```python
from build123d import *

# Parameters (mm, degrees)
CYLINDER_R           = 35
CYLINDER_DEPTH       = 100
CYLINDER_PITCH_ANGLE = 90
BOX003_W             = 170
BOX003_H             = 169
BOX003_DEPTH         = 74
BOX001_W             = 170
BOX001_H             = 190
BOX001_DEPTH         = 166
BOX_W                = 180
BOX_H                = 200
BOX_DEPTH            = 350
BOX002_W             = 180
BOX002_H             = 80
BOX002_DEPTH         = 28
FILLET_R             = 10
FILLET001_R          = 10
FILLET002_R          = 10
FILLET003_R          = 10
FILLET004_R          = 10
FILLET005_R          = 15
FILLET006_R          = 10


with BuildPart() as cylinder:
    # Cylinder → Cylinder (new body)
    with BuildSketch(Plane.XY):
        Circle(CYLINDER_R)
    extrude(amount=CYLINDER_DEPTH)


with BuildPart() as cylinder_1:
    # Cylinder pitch: moved
    add(cylinder.part.rotate(Axis((0, 0, 0), (0, 1, 0)), CYLINDER_PITCH_ANGLE))


with BuildPart() as cylinder_2:
    # Cylinder placement: moved
    add(cylinder_1.part.moved(Location((43, 100, 70))))


with BuildPart() as cube003:
    # Box003 → Box003 (new body)
    with BuildSketch(Plane(origin=(5, -68, 5), x_dir=(1, 0, 0), z_dir=(0, 0, 1))):
        with Locations((85, 84.5)):
            Rectangle(BOX003_W, BOX003_H)
    extrude(amount=BOX003_DEPTH)


with BuildPart() as cube001:
    # Box001 → Box001 (new body)
    with BuildSketch(Plane(origin=(5, 5, 187), x_dir=(1, 0, 0), z_dir=(0, 0, 1))):
        with Locations((85, 95)):
            Rectangle(BOX001_W, BOX001_H)
    extrude(amount=BOX001_DEPTH)


with BuildPart() as cone:
    # Cone → Cone (revolve)
    with BuildSketch(Plane(origin=(90, 100, 88), x_dir=(1, 0, 0), z_dir=(0, -1, 0))):
        Polygon((0, 0), (40, 0), (85, 100), (0, 100), align=None)
    revolve(axis=Axis((90, 100, 88), (0, 0, 1)))


with BuildPart() as cut001:
    # Box → Box (new body)
    with BuildSketch(Plane.XY):
        with Locations((90, 100)):
            Rectangle(BOX_W, BOX_H)
    extrude(amount=BOX_DEPTH)

    # Cut: cut Cone
    add(cone.part, mode=Mode.SUBTRACT)

    # Cut001: cut Cube001
    add(cube001.part, mode=Mode.SUBTRACT)


with BuildPart() as fillet006:
    # Box002 → Box002 (new body)
    with BuildSketch(Plane(origin=(0, -75, 0), x_dir=(1, 0, 0), z_dir=(0, 0, 1))):
        with Locations((90, 40)):
            Rectangle(BOX002_W, BOX002_H)
    extrude(amount=BOX002_DEPTH)

    # Fusion: union Cut001
    add(cut001.part)

    # Cut002: cut Cube003
    add(cube003.part, mode=Mode.SUBTRACT)

    # Cut003: cut Cylinder
    add(cylinder_2.part, mode=Mode.SUBTRACT)

    # Fillet
    fillet_edges = [fillet006.edges().sort_by_distance(p)[0] for p in [
        (180, 200, 175),
    ]]
    fillet(fillet_edges, radius=FILLET_R)

    # Fillet001
    fillet001_edges = [fillet006.edges().sort_by_distance(p)[0] for p in [
        (0, 200, 175),
    ]]
    fillet(fillet001_edges, radius=FILLET001_R)

    # Fillet002
    fillet002_edges = [fillet006.edges().sort_by_distance(p)[0] for p in [
        (180, -75, 14),
    ]]
    fillet(fillet002_edges, radius=FILLET002_R)

    # Fillet003
    fillet003_edges = [fillet006.edges().sort_by_distance(p)[0] for p in [
        (0, -75, 14),
    ]]
    fillet(fillet003_edges, radius=FILLET003_R)

    # Fillet004
    fillet004_edges = [fillet006.edges().sort_by_distance(p)[0] for p in [
        (5.45, 100, 187),
    ]]
    fillet(fillet004_edges, radius=FILLET004_R)

    # Fillet005
    fillet005_edges = [fillet006.edges().sort_by_distance(p)[0] for p in [
        (93, 101, 35.014289),
    ]]
    fillet(fillet005_edges, radius=FILLET005_R)

    # Fillet006
    fillet006_edges = [fillet006.edges().sort_by_distance(p)[0] for p in [
        (90, 0, 79),
    ]]
    fillet(fillet006_edges, radius=FILLET006_R)


solid = fillet006.part
```
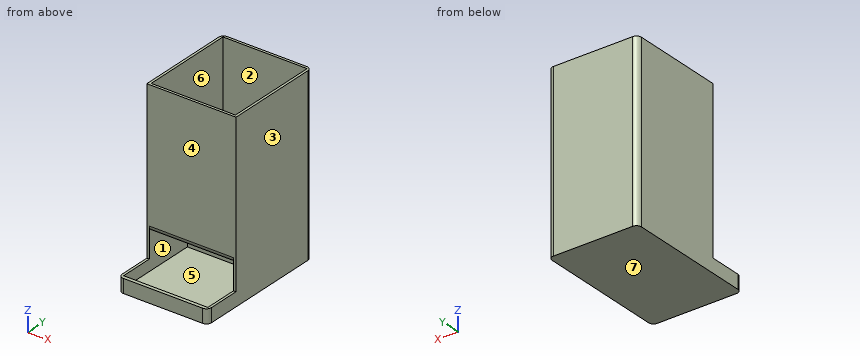
Could you check a few things on this model? Use its own coordinates, in mm. Face numbers are marked on the shaded views. A direction names the side the tool comes from. Give positions to 0.01 mm unless a question says otherwise; leave off trailing zeros. Loops run counter-clockwise (first coordinate to the right, second up) from the corner with the lowest first, then second, coordinate; pieces in that order, holes last. Notation, with made-up numbers: (65, 65.25) -> (107, 65.25) arc R11 cw to (107, 74.25) -> close; hole circle Ø4 at (-18, 67.25). An arc over 180 degrees is marked (long way). Put each result on its own line as item: value.
(1) Imagine slicing it at D-D on z = 209. Write out the boundary of the cut face in (x, y), plus the area to 3 significant figures.
Computed:
outline: (0, 0) -> (180, 0) -> (180, 190) arc R10 ccw to (170, 200) -> (10, 200) arc R10 ccw to (0, 190) -> close; hole (5, 5) -> (175, 5) -> (175, 195) -> (5, 195) -> close
area: 3,660 mm^2
(2) Imagine slicing it at A-A on x = 90. Write out the boundary of the cut face in (y, z), plus the area to 3 significant figures.
Computed:
outline: (-75, 0) -> (200, 0) -> (200, 350) -> (195, 350) -> (195, 187) -> (191.02, 187) arc R10 ccw to (181.9, 181.1) -> (140, 88) -> (130.02, 88) arc R35 cw to (111.2, 36.84) arc R15 ccw to (101, 22.63) -> (101, 5) -> (-68, 5) -> (-68, 28) -> (-75, 28) -> close; (0, 89) arc R10 ccw to (10, 79) -> (66.18, 79) arc R35 cw to (69.98, 88) -> (60, 88) -> (18.1, 181.1) arc R10 ccw to (8.98, 187) -> (5, 187) -> (5, 350) -> (0, 350) -> close
area: 17,900 mm^2
(3) Please list where these lines run through material, in increasing order: probe 1 along Y at (x, z) = (164, 205); probe 2 along X at (y, z) = (172, 240.5); probe 3 along X at (y, z) = (108, 47). Write a range as [from, to].
Computed:
probe 1: [0, 5], [195, 200]
probe 2: [0, 5], [175, 180]
probe 3: [0, 43], [143, 180]
(4) I'm going to push flat-ended pins straight in: pin 1 Ø5 at (x, y) = (83.5, 66) entering from +Z; pin 2 Ø1 at (x, y) = (135, 94) entering from +Z; pin 3 Ø8 at (x, z) = (160, 232.5) entering from -Y. Where does each tip first touch, or does it pass through?
Computed:
pin 1: z = 88
pin 2: z = 5
pin 3: y = 0
(5) For the marked faces 1, 2, 3 and 4, which set-ups out of +Z, -Z, +X, -X, +Y, -Y let a thin tool reach every point of the face, with its end or its side?
Computed:
face 1: none
face 2: +Z
face 3: +Z, -Z, +X, +Y, -Y
face 4: +Z, +X, -X, -Y
(6) Imagine slicing it at C-C on z = 70. Write out the boundary of the cut face in (x, y).
Computed:
outline: (0, 0) -> (5, 0) -> (5, 101) -> (43, 101) -> (43, 135) -> (143, 135) -> (143, 101) -> (175, 101) -> (175, 0) -> (180, 0) -> (180, 190) arc R10 ccw to (170, 200) -> (10, 200) arc R10 ccw to (0, 190) -> close
(7) Thinking about a two-plate mould opening in Z: for the marked faces 5, 6 and 7, which applies, pulls with the +Z half, pulls with the -Z half, needs draft (parallel to the pull), parting line crosses it, or undercut?
Computed:
face 5: undercut
face 6: needs draft
face 7: pulls with the -Z half
(8) Imagine slicing it at B-B on z = 152. Write out the boundary of the cut face in (x, y).
Computed:
outline: (0, 0) -> (180, 0) -> (180, 190) arc R10 ccw to (170, 200) -> (10, 200) arc R10 ccw to (0, 190) -> close; hole circle Ø137.6 at (90, 100)
